Model file for the job. Use its own axes, mm. Round coordinates to 2 decimals unless told otherwise and drop trailing zeros. Order: outer loops, then holes, each group sorted by start corner. A loop starts at its lowest first (then second) coordinate and runs counter-clockwise, first axis right, second up. Notation, with made-up numbers: M 48.5,37 L 83.5,37 A22 ccw 83.5,60 Z; hole C -12.5,67 d11. An arc over 180 degrees is marked long. Return JSON: item names as keys, results as strings. Group by question number.
Item 1: Slice it at A-A on x = 0. Write the cut outline in (y, z).
Item 2: Slice it at B-B on x = -22.6. Write the cut outline in (y, z).
Item 3: Pin check, flat tip, straight feed: pin 1 Ø2.5 at (x, y) = (47.5, -54.43) entering from -Z. Stop position of the tip, or through.
Item 4: Probe line 1 along Y through (x, z) = (53.5, 0.85); line 2 along Y through (x, z) = (22.6, 2.35); line 3 along Y through (x, z) = (-51, 2.45). List the from-to ranges inside material, lowest first.
Item 5: Pull direction Y, two halves, no side cores. Call faces 1 (the face through (45.29, -45.47, 1.48)), 2 (the face through (-26, 26, 0)), 3 (the face through (-1, 57.5, 1)): pulls with the +Y half, pulls with the -Y half, needs draft (parallel to the pull), parting line crosses it, or undercut.
Item 6: Slice it at D-D on z = 1.15. Give the number of separate pieces and of enclosed holes in the cut face, then the cut area to 3 significant figures.
Item 7: Slice it at C-C on y = -28.5. Write the cut outline in (x, z), then the cut area to 3 significant figures.
from build123d import *

# Parameters (mm, degrees)
SKETCH_1_W            = 115
SKETCH_1_H            = 115
SKETCH_1_R            = 30
SKETCH_1_R_2          = 3
EXTRUDE_1_DEPTH       = 3
CUT_EXTRUDE_2_DEPTH   = 82.372599811
MIRROR_4_COPY_1_DEPTH = 82.372599811
SKETCH_4_R            = 4.25
CUT_EXTRUDE_3_DEPTH   = 3


with BuildPart() as part:
    # 草图1 → 凸台-拉伸1 (new body)
    with BuildSketch(Plane.XY):
        Rectangle(SKETCH_1_W, SKETCH_1_H)
        Circle(SKETCH_1_R, mode=Mode.SUBTRACT)
        with Locations((-47.5, 47.5)):
            Circle(SKETCH_1_R_2, mode=Mode.SUBTRACT)
        with Locations((47.5, 47.5)):
            Circle(SKETCH_1_R_2, mode=Mode.SUBTRACT)
        with Locations((47.5, -47.5)):
            Circle(SKETCH_1_R_2, mode=Mode.SUBTRACT)
        with Locations((-47.5, -47.5)):
            Circle(SKETCH_1_R_2, mode=Mode.SUBTRACT)
    extrude(amount=EXTRUDE_1_DEPTH)

    # 草图3 → 切除-拉伸2 (cut, through all)
    with BuildSketch(Plane.XY.offset(3)):
        with BuildLine():
            ThreePointArc((-52, 44.035898385), (-52.200961894, 44.785898385), (-52.75, 45.334936491))
            Line((-52.75, 45.334936491), (-53.5, 44.035898385))
            Line((-53.5, 44.035898385), (-52, 44.035898385))
        make_face()
        with BuildLine():
            Line((-53.5, 44.035898385), (-52.75, 45.334936491))
            ThreePointArc((-52.75, 45.334936491), (-54.799038106, 43.285898385), (-52, 44.035898385))
            Line((-52, 44.035898385), (-53.5, 44.035898385))
        make_face()
        with BuildLine():
            ThreePointArc((-40, 44.035898385), (-40.75, 45.334936491), (-42.25, 45.334936491))
            Line((-42.25, 45.334936491), (-41.5, 44.035898385))
            Line((-41.5, 44.035898385), (-43, 44.035898385))
            ThreePointArc((-43, 44.035898385), (-41.5, 42.535898385), (-40, 44.035898385))
        make_face()
        with BuildLine():
            Line((-41.5, 44.035898385), (-42.25, 45.334936491))
            ThreePointArc((-42.25, 45.334936491), (-42.799038106, 44.785898385), (-43, 44.035898385))
            Line((-43, 44.035898385), (-41.5, 44.035898385))
        make_face()
        with BuildLine():
            Line((-46.75, 53.129165125), (-47.5, 54.42820323))
            Line((-47.5, 54.42820323), (-48.25, 53.129165125))
            ThreePointArc((-48.25, 53.129165125), (-47.5, 52.92820323), (-46.75, 53.129165125))
        make_face()
        with BuildLine():
            Line((-48.25, 53.129165125), (-47.5, 54.42820323))
            Line((-47.5, 54.42820323), (-46.75, 53.129165125))
            ThreePointArc((-46.75, 53.129165125), (-46.200961894, 53.67820323), (-46, 54.42820323))
            ThreePointArc((-46, 54.42820323), (-48.25, 55.727241336), (-48.25, 53.129165125))
        make_face()
    cut_extrude_2 = extrude(amount=-CUT_EXTRUDE_2_DEPTH, mode=Mode.SUBTRACT)

    # 镜向3: 切除-拉伸2 across plane
    add(cut_extrude_2.mirror(Plane(origin=(0, 0, 0), x_dir=(0, 0, 1), z_dir=(1, 0, 0))), mode=Mode.SUBTRACT)

    # 镜向4: 切除-拉伸2 across plane
    add(cut_extrude_2.mirror(Plane.ZX), mode=Mode.SUBTRACT)

    # 镜向4 copy 1 sketch → 镜向4 copy 1 (cut, through all)
    with BuildSketch(Plane(origin=(0, 0, 3), x_dir=(-1, 0, 0), z_dir=(0, 0, 1))):
        with BuildLine():
            ThreePointArc((-52, 44.035898385), (-52.200961894, 44.785898385), (-52.75, 45.334936491))
            Line((-52.75, 45.334936491), (-53.5, 44.035898385))
            Line((-53.5, 44.035898385), (-52, 44.035898385))
        make_face()
        with BuildLine():
            Line((-53.5, 44.035898385), (-52.75, 45.334936491))
            ThreePointArc((-52.75, 45.334936491), (-54.799038106, 43.285898385), (-52, 44.035898385))
            Line((-52, 44.035898385), (-53.5, 44.035898385))
        make_face()
        with BuildLine():
            ThreePointArc((-40, 44.035898385), (-40.75, 45.334936491), (-42.25, 45.334936491))
            Line((-42.25, 45.334936491), (-41.5, 44.035898385))
            Line((-41.5, 44.035898385), (-43, 44.035898385))
            ThreePointArc((-43, 44.035898385), (-41.5, 42.535898385), (-40, 44.035898385))
        make_face()
        with BuildLine():
            Line((-41.5, 44.035898385), (-42.25, 45.334936491))
            ThreePointArc((-42.25, 45.334936491), (-42.799038106, 44.785898385), (-43, 44.035898385))
            Line((-43, 44.035898385), (-41.5, 44.035898385))
        make_face()
        with BuildLine():
            Line((-46.75, 53.129165125), (-47.5, 54.42820323))
            Line((-47.5, 54.42820323), (-48.25, 53.129165125))
            ThreePointArc((-48.25, 53.129165125), (-47.5, 52.92820323), (-46.75, 53.129165125))
        make_face()
        with BuildLine():
            Line((-48.25, 53.129165125), (-47.5, 54.42820323))
            Line((-47.5, 54.42820323), (-46.75, 53.129165125))
            ThreePointArc((-46.75, 53.129165125), (-46.200961894, 53.67820323), (-46, 54.42820323))
            ThreePointArc((-46, 54.42820323), (-48.25, 55.727241336), (-48.25, 53.129165125))
        make_face()
    extrude(amount=-MIRROR_4_COPY_1_DEPTH, mode=Mode.SUBTRACT)

    # 草图4 → 切除-拉伸3 (cut)
    with BuildSketch(Plane.XY.offset(3)):
        with Locations((-22.6, 48)):
            Circle(SKETCH_4_R)
        with Locations((-48, 22.6)):
            Circle(SKETCH_4_R)
        with Locations((22.6, 48)):
            Circle(SKETCH_4_R)
        with Locations((48, 22.6)):
            Circle(SKETCH_4_R)
        with Locations((48, -22.6)):
            Circle(SKETCH_4_R)
        with Locations((22.6, -48)):
            Circle(SKETCH_4_R)
        with Locations((-48, -22.6)):
            Circle(SKETCH_4_R)
        with Locations((-22.6, -48)):
            Circle(SKETCH_4_R)
    extrude(amount=-CUT_EXTRUDE_3_DEPTH, mode=Mode.SUBTRACT)


solid = part.part
Output values:
{
 "1": {"outline": "M -57.5,0 L -30,0 L -30,3 L -57.5,3 Z; M 30,0 L 57.5,0 L 57.5,3 L 30,3 Z"},
 "2": {"outline": "M -57.5,0 L -52.25,0 L -52.25,3 L -57.5,3 Z; M -43.75,0 L -19.73,0 L -19.73,3 L -43.75,3 Z; M 19.73,0 L 43.75,0 L 43.75,3 L 19.73,3 Z; M 52.25,0 L 57.5,0 L 57.5,3 L 52.25,3 Z"},
 "3": {"pin 1": "through"},
 "4": {"line 1": "-57.5 to -45.54, -42.54 to 42.54, 45.54 to 57.5", "line 2": "-57.5 to -52.25, -43.75 to -19.73, 19.73 to 43.75, 52.25 to 57.5", "line 3": "-57.5 to -25.61, -19.59 to 19.59, 25.61 to 57.5"},
 "5": {"face 1": "undercut", "face 2": "needs draft", "face 3": "pulls with the +Y half"},
 "6": {"separate pieces": "1", "enclosed holes": "25", "area": "9,750 mm²"},
 "7": {"outline": "M -57.5,0 L -9.37,0 L -9.37,3 L -57.5,3 Z; M 9.37,0 L 57.5,0 L 57.5,3 L 9.37,3 Z", "area": "289 mm²"}
}
